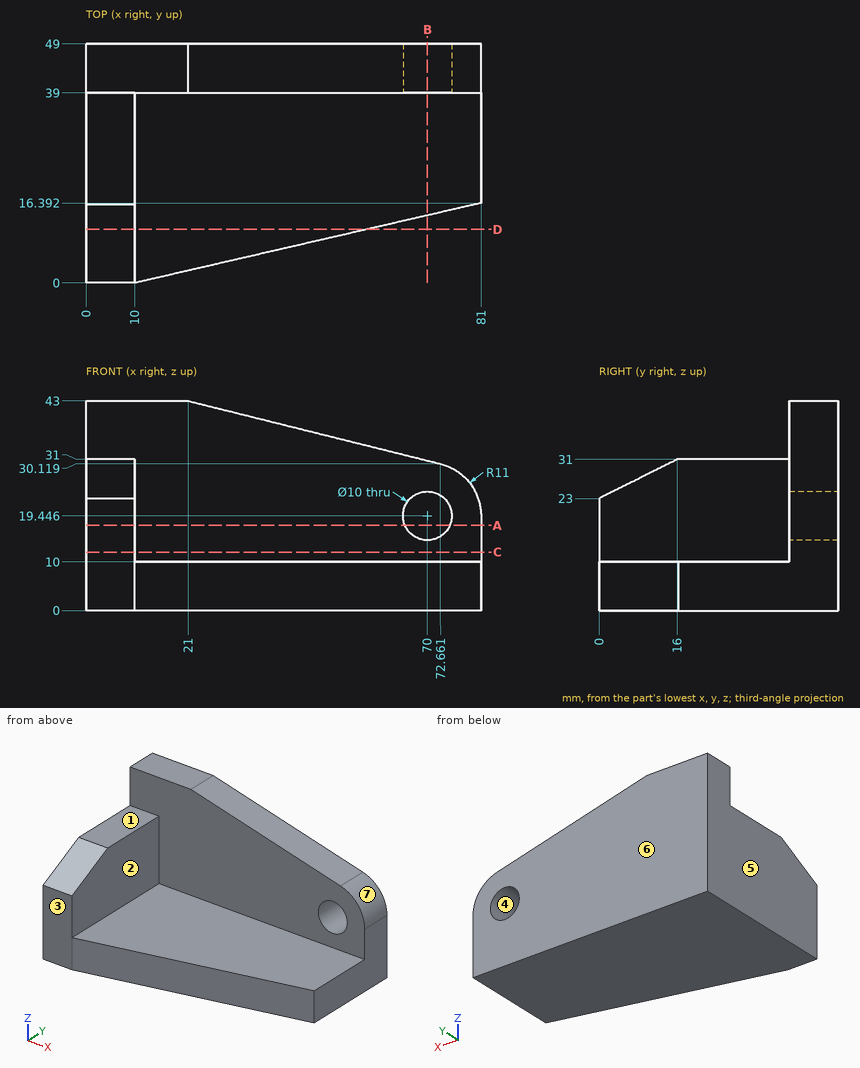
Source: three-view drawing plus pictorial views. Frame: mm from the lowest corner of the part. A direction names the side the tool comes from. Coordinates: 2 decimals unless noted, no trailing zeros. Loops run counter-clockwise (first coordinate to the right, second up) from the corner with the lowest first, then second, coordinate; pieces in that order, holes last. Notation, with made-up numbers: (-13.5, 85) -> (44.5, 85) arc R31 ccw to (44.5, 122) -> close; hole circle Ø1 at (0, 34). An arc over 180 degrees is marked (long way). Write each question's results on one line, items separated by ' | '. Start each with the question number.
Q1. Pull-direction query (X, two-part tool) for the marked faces 4, 5, 6 and 7; classes: released by +X, released by -X, zero draft, split by the parting line, or undercut.
Q2. Section A-A, the plane z = 17.5. Return the cut outline in (x, y) (1 decimal), plus the area to 3 significant figures.
Q3. Pin query (flat end, axial travel): pin 1 (5 mm diameter, centred on y = 38.5, z = 14.5, fed in from -X); pin 2 (6.5 mm diameter, centred on y = 13.5, z = 16.5, fed in from +X); pin 3 (19.5 mm diameter, centred on x = 53.5, y = 17.5, fed in from +Z); pin 4 (2 mm diameter, centred on x = 40.5, z = 24.5, fed in from -Y). Return the tip coordinate at first contact, or that it passes through.
Q4. Ray query, line 1 (Z direction, x = 29, y = 8); line 2 (Y direction, x = 27.5, z = 25.5). Return the intervals inside material, ascending. Write a range as from..to.
Q5. Section C-C, the plane z = 12. Return the cut outline in (x, y), plus the area to 3 significant figures.
Q6. Section B-B, the plane x = 70. Return the cut outline in (y, z).
Q7. Section D-D, the plane y = 11. Return the cut outline in (x, z).
Q8. Reachability of the marked faces 1, 2 and 3 from +Z, -Z, +X, -X, +Y, -Y: full face, straight path, thin tool, end or side. Return the list, or none.
Found:
1) face 4: undercut | face 5: released by -X | face 6: zero draft | face 7: released by +X
2) outline: (0, 0) -> (10, 0) -> (10, 39) -> (65.4, 39) -> (65.4, 49) -> (0, 49) -> close; (74.6, 39) -> (81, 39) -> (81, 49) -> (74.6, 49) -> close | area: 1,110 mm2
3) pin 1: x = 0 | pin 2: x = 10 | pin 3: z = 10 | pin 4: y = 39
4) line 1: 0..10 | line 2: 39..49
5) outline: (0, 0) -> (10, 0) -> (10, 39) -> (81, 39) -> (81, 49) -> (0, 49) -> close | area: 1,200 mm2
6) outline: (13.85, 0) -> (49, 0) -> (49, 14.45) -> (39, 14.45) -> (39, 10) -> (13.85, 10) -> close; (39, 24.45) -> (49, 24.45) -> (49, 30.78) -> (39, 30.78) -> close
7) outline: (0, 0) -> (57.65, 0) -> (57.65, 10) -> (10, 10) -> (10, 28.5) -> (0, 28.5) -> close
8) face 1: +Z, +X, -X, -Y | face 2: +Z, +X, -Y | face 3: +Z, -Z, +X, -X, -Y
